Here's how the part is built. I have some questions about the finished solid (model axes, mm). A direction names the side the tool comes from. Round coordinates to 2 decimals unless told otherwise and drop trailing zeros. Loops run counter-clockwise (first coordinate to the right, second up) from the corner with the lowest first, then second, coordinate; pieces in that order, holes last. Notation, with made-up numbers: M 45,0.5 L 54,0.5 A12 cw 54,23.5 Z; hole C 18.25,-18 d7. An arc over 180 degrees is marked long. Answer as a JSON object with one key per item and string values.
from build123d import *

# Parameters (mm, degrees)
BOSS_EXTRUDE1_DEPTH = 35
BOSS_EXTRUDE2_DEPTH = 10
FILLET1_R           = 3
FILLET3_R           = 3
BOSS_EXTRUDE3_START = 4
BOSS_EXTRUDE3_DEPTH = 4
SKETCH4_R           = 8
CUT_EXTRUDE7_DEPTH  = 54.020962835
CUT_EXTRUDE7_DRAFT  = -0.4


# Read off the part's stored shape, not the designer's step: Boss-Extrude2
with BuildPart() as part:
    # Sketch1 → Boss-Extrude1 (new body)
    with BuildSketch(Plane(origin=(0, 0, 0), x_dir=(0, 0, -1), z_dir=(1, 0, 0))):
        with BuildLine():
            Line((-9, 0), (-16.35, 0))
            Line((-16.35, 0), (-23.35, 0))
            Line((-23.35, 0), (-23.35, -4))
            Line((-23.35, -4), (-15, -4))
            ThreePointArc((-15, -4), (0, -15.524174696), (15, -4))
            Line((15, -4), (23.35, -4))
            Line((23.35, -4), (23.35, 0))
            Line((23.35, 0), (16.35, 0))
            Line((16.35, 0), (9, 0))
            Line((9, 0), (-9, 0))
        make_face()
    extrude(amount=BOSS_EXTRUDE1_DEPTH)

    # Boss-Extrude2 outline → Boss-Extrude2 (add)
    with BuildSketch(Plane.ZY):
        with BuildLine():
            Line((15.524174696, 0), (-15.524174696, 0))
            ThreePointArc((-15.524174696, 0), (0, -15.524174696), (15.524174696, 0))
        make_face()
    extrude(amount=BOSS_EXTRUDE2_DEPTH)

    # Fillet1
    fillet1_edges = [part.edges().sort_by_distance(p)[0] for p in [
        (35, -2, 23.35),
    ]]
    fillet(fillet1_edges, radius=FILLET1_R)

    # Fillet3
    fillet3_edges = [part.edges().sort_by_distance(p)[0] for p in [
        (35, -2, -23.35),
    ]]
    fillet(fillet3_edges, radius=FILLET3_R)

    # Sketch3 → Boss-Extrude3 (add)
    with BuildSketch(Plane.ZY.offset(BOSS_EXTRUDE3_START)):
        with BuildLine():
            Line((-15.524174696, 0), (-23.35, 0))
            Line((-23.35, 0), (-23.35, -4))
            Line((-23.35, -4), (-15, -4))
            ThreePointArc((-15, -4), (-15.392573216, -2.017099348), (-15.524174696, 0))
        make_face()
        with BuildLine():
            Line((23.35, -4), (15, -4))
            ThreePointArc((15, -4), (15.392573216, -2.017099348), (15.524174696, 0))
            Line((15.524174696, 0), (23.35, 0))
            Line((23.35, 0), (23.35, -4))
        make_face()
    extrude(amount=-BOSS_EXTRUDE3_DEPTH)


with BuildPart() as cut_extrude7_tool:
    # Sketch4 → Cut-Extrude7 (with draft: the straight prism first)
    with BuildSketch(Plane.ZY.offset(10)):
        Circle(SKETCH4_R)
    extrude(amount=-CUT_EXTRUDE7_DEPTH)
    # Cut-Extrude7: the draft: its side faces are tilted about the plane it starts from
    cut_extrude7_sides = [cut_extrude7_tool.faces().sort_by_distance(p)[0] for p in [
        (17.010481418, 0, -8),
    ]]
    draft(cut_extrude7_sides, Plane.ZY.offset(10), CUT_EXTRUDE7_DRAFT)


with BuildPart() as part_1:
    add(part.part)

    # Cut-Extrude7: cut by cut_extrude7_tool
    add(cut_extrude7_tool.part, mode=Mode.SUBTRACT)


solid = part_1.part
Item 1: If we mould it in two halves opening along Z, with no side actions, what happens to faces 1 (the face through (12.185, -7.843, -0.173)), 2 (the face through (14, -2, -23.35)), 3 (the face through (15, -4, -19))? For each: pulls with the +Z half, pulls with the -Z half, needs draft (parallel to the pull), parting line crosses it, or undercut.
Resolved:
{"face 1": "undercut", "face 2": "pulls with the -Z half", "face 3": "needs draft"}
Item 2: I want a section at D-D, the plane x = 28. Please give me the cut outline in (y, z), then the cut area to 3 significant figures.
Resolved:
{"outline": "M -4,-23.35 L 0,-23.35 L 0,-7.73 A7.73 cw 0,7.73 L 0,23.35 L -4,23.35 L -4,15 A15.52 ccw -4,-15 Z", "area": "349 mm²"}
Item 3: On a 3-axis mill with a long thin cutter (end or side, diameter ignored), from which of +Z, -Z, +X, -X, +Y, -Y can I reach the whole of each face in a straight line? I mean faces 4 (the face through (12, 0, 16)), 5 (the face through (15, -4, 19)). Say none if no direction works.
Resolved:
{"face 4": "+Z, -Z, +X, -X, +Y", "face 5": "+Z, +X, -X, -Y"}
Item 4: Please list where these lines run through material, in increasing order: probe 1 along Z at (x, y) = (7, -3.25); probe 2 along Z at (x, y) = (11, -5.25); probe 3 along Y at (x, z) = (6, -18). Write a range as from..to.
Resolved:
{"probe 1": "-23.35..-7.18, 7.18..23.35", "probe 2": "-14.61..-5.84, 5.84..14.61", "probe 3": "-4..0"}
Item 5: I'm going to push flat-ended pins straight in: pin 1 Ø12 at (x, z) = (3.5, 7.5) entering from +Y; pin 2 Ø10 at (x, z) = (-2, -8) entering from -Y; pin 3 Ø2 at (y, z) = (-2, 19.5) entering from -X; pin 4 Ø6 at (x, y) = (20.5, -11.5) entering from -Z. Where does each tip first touch, or does it pass through?
Resolved:
{"pin 1": "y = 0", "pin 2": "y = -15.23", "pin 3": "x = -4", "pin 4": "z = -12.99"}
Item 6: I want a section at B-B, the plane y = -10.75. Please give me the cut outline in (x, z).
Resolved:
{"outline": "M -10,-11.2 L 35,-11.2 L 35,11.2 L -10,11.2 Z"}
Item 7: I want a section at C-C, the plane z = -19.5. Please give me the cut outline in (x, y), then the cut area to 3 significant figures.
Resolved:
{"outline": "M -4,-4 L 35,-4 L 35,0 L -4,0 Z", "area": "156 mm²"}
Item 8: I want a section at A-A, the plane x = 21.5. Please give me the cut outline in (y, z).
Resolved:
{"outline": "M -4,-23.35 L 0,-23.35 L 0,-7.78 A7.78 cw 0,7.78 L 0,23.35 L -4,23.35 L -4,15 A15.52 ccw -4,-15 Z"}
